Work out the finished part from the listing and answer in its coordinate system (mm). Face numbers are marked on the shaded views. Give positions to 0.01 mm unless a question says otherwise; leave off trailing zeros. Write each loop counter-clockwise with the first axis right and the second up, starting at its lowest first coordinate (ties: lowest second). Pieces come first, ordered by that corner, then holes. Notation, with made-up numbers: (83, 63) - (97, 63) arc R35 ccw to (97, 102) - close; hole circle Ø10 at (74.25, 25). An arc over 180 degrees is marked (long way). Write item = value, one per line.
from build123d import *

# Parameters (mm, degrees)
F2_R = 2


with BuildPart() as f1:
    # F0 (on Front) → F1 (revolve)
    with BuildSketch(Plane.XZ):
        Polygon((17.658173, 7.978278), (1.658173, 7.978278), (0, 7.978278), (0, 6.885595), (1.502076, 6.885595), (16.409393, 6.885595), (16.409393, -5.914406), (18.672808, -5.914406), (18.672808, -4.197333), (17.658173, -3.182699), align=None)
    revolve(axis=Axis((0, 0, 7.431936), (0, 0, 1)))

    # F2
    f2_edges = [f1.edges().sort_by_distance(p)[0] for p in [
        (-17.658173, 0, 7.978278),
    ]]
    fillet(f2_edges, radius=F2_R)


solid = f1.part
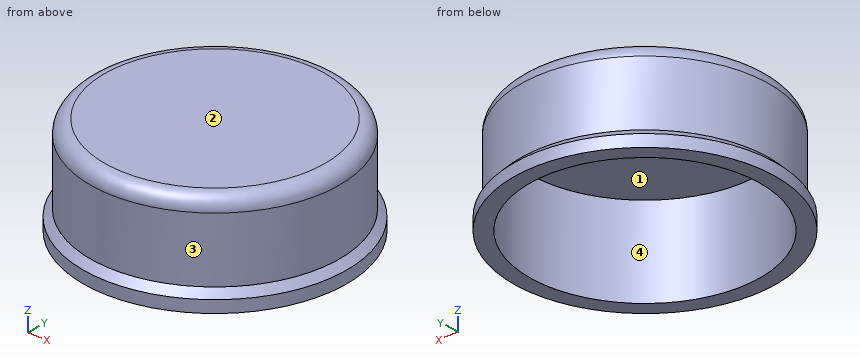
1. Find section A-A, the plane y = 0. Give the vertices of the cut face in (x, z), then the cut area to 3 significant figures.
Solution:
outline = (-18.67, -5.91) - (-16.41, -5.91) - (-16.41, 6.89) - (16.41, 6.89) - (16.41, -5.91) - (18.67, -5.91) - (18.67, -4.2) - (17.66, -3.18) - (17.66, 5.98) arc R2 ccw to (15.66, 7.98) - (-15.66, 7.98) arc R2 ccw to (-17.66, 5.98) - (-17.66, -3.18) - (-18.67, -4.2) - close
area = 73.4 mm^2
2. Find section B-B, the plane z = 3.25. Give the vertices of the cut face in (x, y).
Solution:
outline = circle Ø35.32 at (0, 0); hole circle Ø32.82 at (0, 0)
3. For a pull along X with two mould halves and no side action, classify the marked faces 1, 2, 3 and 4 as pulls with the +X half, pulls with the -X half, needs draft (parallel to the pull), parting line crosses it, or undercut.
Solution:
face_1 = undercut
face_2 = needs draft
face_3 = parting line crosses it
face_4 = undercut
4. Straight lines are drawn through the part: line 1 (Y direction, x = 0, z = 3.25); line 2 (Y direction, x = 9.5, z = -2.75); line 3 (Z direction, x = -3.5, y = -7). For each, find the intervals that lie inside material, in ascending order.
Solution:
line_1 = -17.66 to -16.41, 16.41 to 17.66
line_2 = -14.88 to -13.38, 13.38 to 14.88
line_3 = 6.89 to 7.98
5. Given pin 1 (2 mm diameter, centred on y = 14, z = 5, fed in from -X); pin 2 (2 mm diameter, centred on y = -3.5, z = -2, fed in from +X); pin 3 (3 mm diameter, centred on x = -14.5, y = 12.5, fed in from -Z); pin 4 (10 mm diameter, centred on x = 4.5, y = -4.5, fed in from -Z), each flat-ended and moving along its own axis, determine where each tip first touches the part or whether it passes through.
Solution:
pin_1 = -11.95
pin_2 = 17.48
pin_3 = -5.91
pin_4 = 6.89
